from build123d import *

# Parameters (mm, degrees)
SKETCH_1_W                = 230
SKETCH_1_H                = 150
EXTRUDE_1_DEPTH           = 10
CHAMFER_1_SIZE            = 1
F_5_0MM_DOWEL_HOLE1_D     = 5
F_5_0MM_DOWEL_HOLE1_DEPTH = 10
F_5_0MM_DOWEL_HOLE1_TIP   = 1.502151548


with BuildPart() as part:
    # Эскиз1 → Бобышка-Вытянуть1 (new body)
    with BuildSketch(Plane(origin=(0, 0, 0), x_dir=(1, 0, 0), z_dir=(0, 1, 0))):
        Rectangle(SKETCH_1_W, SKETCH_1_H)
    extrude(amount=-EXTRUDE_1_DEPTH)

    # Фаска1
    chamfer_1_edges = [part.edges().sort_by_distance(p)[0] for p in [
        (0, 0, 75),
        (-115, 0, 0),
        (0, 0, -75),
        (115, 0, 0),
    ]]
    chamfer(chamfer_1_edges, length=CHAMFER_1_SIZE)

    # Ø5.0mm Dowel Hole1
    with Locations(Plane(origin=(0, 0, 0), x_dir=(-1, 0, 0), z_dir=(0, 1, 0))):
        with Locations((0, 37.5), (0, -37.5)):
            Hole(F_5_0MM_DOWEL_HOLE1_D / 2, depth=F_5_0MM_DOWEL_HOLE1_DEPTH)
            with Locations((0, 0, -(F_5_0MM_DOWEL_HOLE1_DEPTH + F_5_0MM_DOWEL_HOLE1_TIP / 2))):  # 118° drill point
                Cone(0, F_5_0MM_DOWEL_HOLE1_D / 2, F_5_0MM_DOWEL_HOLE1_TIP, mode=Mode.SUBTRACT)


solid = part.part
Part model, mm, in its own coordinate system. Give positions to 0.01 mm unless a question says otherwise; leave off trailing zeros. Write each loop counter-clockwise with the first axis right and the second up, starting at its lowest first coordinate (ties: lowest second). Pieces come first, ordered by that corner, then holes.
1) Probe L1, parallel to Z at x = 0, y = -6.5; L2, parallel to X at y = -5.75, z = -37.5; L3, parallel to Z at x = -40, y = -0.25. List the from-to ranges inside material, lowest first.
Resolved:
L1: z = -75 to -40, -35 to 35, 40 to 75
L2: x = -115 to -2.5, 2.5 to 115
L3: z = -74.25 to 74.25
2) Pin check, flat tip, straight feed: pin 1 (4 mm diameter, centred on x = 0, z = 37.5, fed in from +Y). Stop position of the tip, or through.
Resolved:
pin 1: passes through
3) Two-plate mould, pull along Z, no slides. Class faces 1 (the face through (-0.54, -5.07, -39.94)), 2 (the face through (-115, -5, 1)), 3 (the face through (-2, -5, -75)): released by +Z, released by -Z, zero draft, split by the parting line, or undercut.
Resolved:
face 1: undercut
face 2: zero draft
face 3: released by -Z
4) Cut at A-A on x = 0. Write the cut outline in (y, z).
Resolved:
outline: (-10, -75) - (-1, -75) - (0, -74) - (0, -40) - (-10, -40) - close; (-10, -35) - (0, -35) - (0, 35) - (-10, 35) - close; (-10, 40) - (0, 40) - (0, 74) - (-1, 75) - (-10, 75) - close
5) Cut at B-B on z = -37.5. Write the cut outline in (x, y).
Resolved:
outline: (-115, -10) - (-2.5, -10) - (-2.5, 0) - (-114, 0) - (-115, -1) - close; (2.5, -10) - (115, -10) - (115, -1) - (114, 0) - (2.5, 0) - close
